Verification items for the finished model (mm, model axes). Round coordinates to 2 decimals unless told otherwise and drop trailing zeros. Order: outer loops, then holes, each group sorted by start corner. A loop starts at its lowest first (then second) coordinate and runs counter-clockwise, first axis right, second up. Notation, with made-up numbers: M 47.5,-1 L 68.5,-1 A30 ccw 68.5,31 Z; hole C -15,-21.5 d11. An arc over 180 degrees is marked long. One line per item, written item: value. Start each with the question number.
from build123d import *

# Parameters (mm, degrees)
SKETCH1_R           = 250
SKETCH1_R_2         = 4.25
SKETCH1_R_3         = 13
BOSS_EXTRUDE1_DEPTH = 9


with BuildPart() as part:
    # Sketch1 → Boss-Extrude1 (new, symmetric)
    with BuildSketch(Plane(origin=(0, 0, 0), x_dir=(1, 0, 0), z_dir=(0, 1, 0))):
        with Locations(Location((0, 0, 0), (0, 0, 270))):
            Circle(SKETCH1_R)
        with Locations(Location((0, 222.5, 0), (0, 0, 270))):
            Circle(SKETCH1_R_2, mode=Mode.SUBTRACT)
        with Locations(Location((111.25, 192.690652342, 0), (0, 0, 270))):
            Circle(SKETCH1_R_2, mode=Mode.SUBTRACT)
        with Locations(Location((192.690652342, 111.25, 0), (0, 0, 270))):
            Circle(SKETCH1_R_2, mode=Mode.SUBTRACT)
        with Locations(Location((222.5, 0, 0), (0, 0, 270))):
            Circle(SKETCH1_R_2, mode=Mode.SUBTRACT)
        with Locations(Location((192.690652342, -111.25, 0), (0, 0, 270))):
            Circle(SKETCH1_R_2, mode=Mode.SUBTRACT)
        with Locations(Location((111.25, -192.690652342, 0), (0, 0, 270))):
            Circle(SKETCH1_R_2, mode=Mode.SUBTRACT)
        with Locations(Location((0, 0, 0), (0, 0, 270))):
            Circle(SKETCH1_R_3, mode=Mode.SUBTRACT)
        with Locations(Location((0, -222.5, 0), (0, 0, 270))):
            Circle(SKETCH1_R_2, mode=Mode.SUBTRACT)
        with Locations(Location((-111.25, -192.690652342, 0), (0, 0, 270))):
            Circle(SKETCH1_R_2, mode=Mode.SUBTRACT)
        with Locations(Location((-192.690652342, -111.25, 0), (0, 0, 270))):
            Circle(SKETCH1_R_2, mode=Mode.SUBTRACT)
        with Locations(Location((-222.5, 0, 0), (0, 0, 270))):
            Circle(SKETCH1_R_2, mode=Mode.SUBTRACT)
        with Locations(Location((-192.690652342, 111.25, 0), (0, 0, 270))):
            Circle(SKETCH1_R_2, mode=Mode.SUBTRACT)
        with Locations(Location((-111.25, 192.690652342, 0), (0, 0, 270))):
            Circle(SKETCH1_R_2, mode=Mode.SUBTRACT)
    extrude(amount=BOSS_EXTRUDE1_DEPTH, both=True)


solid = part.part
1. Draft check along X on faces 1 (the face through (-52, 9, -3)), 2 (the face through (10.99, 0.13, -249.76)), 3 (the face through (-7.91, -0.126, -10.316)). Enter one of: released by +X, released by -X, zero draft, split by the parting line, or undercut.
2. Section check A-A (y = 6). Give the number of separate pieces and of enclosed holes in the cut face, and give its area (3 significant figures).
3. Section check C-C (x = 83). Record the cut outline in (y, z), and give its area (3 significant figures).
4. Section check B-B (z = -70). Record the cut outline in (x, y).
5. Scan lines: line 1 along Z through (x, y) = (190.5, 7.75); line 2 along X through (y, z) = (2.25, -111.25); line 3 along X through (y, z) = (-1.25, -222.5). Record each from-to range of solid material in increasing order.
6. Depth check by flat-ended pin: pin 1 (5 mm diameter, centred on x = 222.5, z = 0, fed in from +Y) (3 decimals); pin 2 (6 mm diameter, centred on x = -115.5, y = -0.5, fed in from +Z); pin 3 (6 mm diameter, centred on y = 5, z = 28.5, fed in from -X); pin 4 (10 mm diameter, centred on x = -60, y = 1, fed in from +Z). Enter the tip coordinate at first touch or a pass-through.
Geometry check:
1. face 1: zero draft
1. face 2: split by the parting line
1. face 3: undercut
2. separate pieces: 1
2. enclosed holes: 13
2. area: 195,000 mm²
3. outline: M -9,-235.82 L 9,-235.82 L 9,235.82 L -9,235.82 Z
3. area: 8,490 mm²
4. outline: M -240,-9 L 240,-9 L 240,9 L -240,9 Z
5. line 1: z = -161.89 to -114.89, -107.61 to 107.61, 114.89 to 161.89
5. line 2: x = -223.88 to -196.94, -188.44 to 188.44, 196.94 to 223.88
5. line 3: x = -113.99 to -4.25, 4.25 to 113.99
6. pin 1: passes through
6. pin 2: stops at z = 223.26
6. pin 3: stops at x = -248.7
6. pin 4: stops at z = 243.87
